Check sheet for the drawn part. Datum: minimum x, y, z corner. Units: mm. Give positions to 0.01 mm unless a question says otherwise; leave off trailing zeros. Order: outer loops, then holes, each group sorted by start corner. A loop starts at its lowest first (then second) coordinate and runs counter-clockwise, first axis right, second up. Notation, with made-up numbers: M 23.5,-27 L 69.5,-27 A20 ccw 69.5,12 Z; hole C 85,75 d3. An arc over 180 degrees is marked long. Answer as CSV lines item,"result". Start each with the question number.
Q1. Section check C-C, the plane x = 178.5. Record the boundary of the cut face in (y, z).
Q2. Section check A-A, the plane z = 23.5. Record the boundary of the cut face in (x, y), then the cut area to 3 significant figures.
Q3. Mould release check, pull along X, two halves, no side actions. Record for the marked faces 1, 2 and 3: +X half, -X half, draft (parallel to the pull), parting line (faces both ways), or undercut.
Q4. Thickness scan on line 1 (X direction, y = 7, z = 10.75); line 2 (X direction, y = 65.5, z = 21.75); line 3 (Z direction, x = 56, y = 56.5). Record the ranges inside material, lowest first.
Q5. Go/stop test with flat-tipped pins: pin 1 (1.5 mm diameter, centred on x = 38, z = 11.5, fed in from +Y); pin 2 (2.5 mm diameter, centred on y = 94, z = 7, fed in from +X); pin 3 (10 mm diameter, centred on x = 39, y = 91.5, fed in from +Z). Record where each tip stops, or that it passes through.
Q6. Section check B-B, the plane y = 39. Record the boundary of the cut face in (x, z), then the cut area to 3 significant figures.
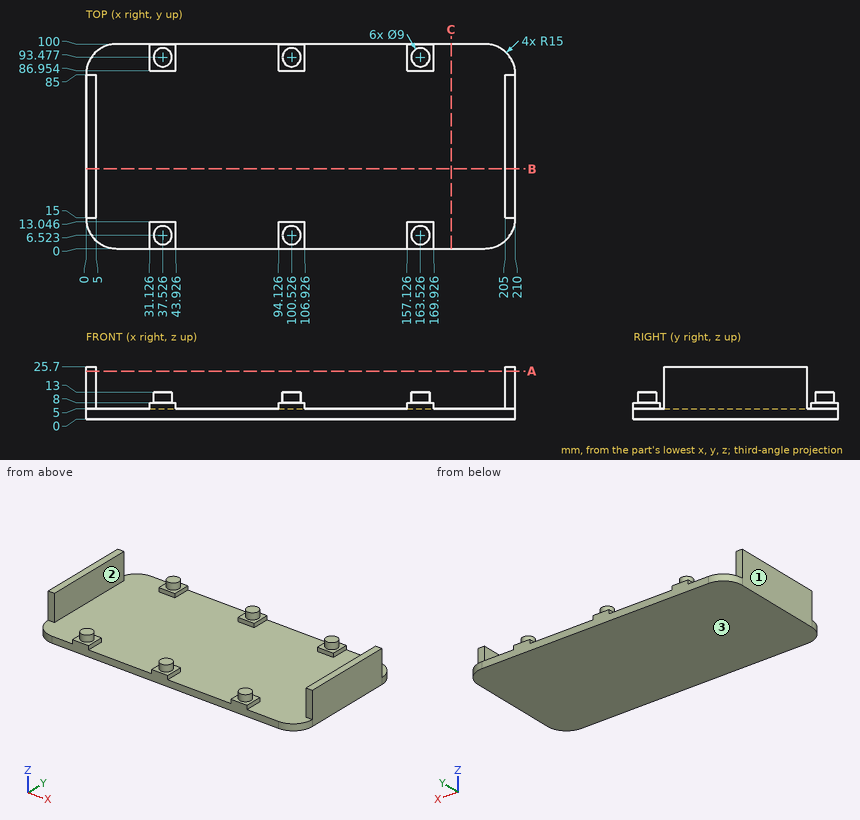
Answer block:
1,outline,"M 0,0 L 100,0 L 100,5 L 0,5 Z"
2,outline,"M 0,15 L 5,15 L 5,85 L 0,85 Z; M 205,15 L 210,15 L 210,85 L 205,85 Z"
2,area,"700 mm2"
3,face 1,"-X half"
3,face 2,"undercut"
3,face 3,"draft"
4,line 1,"x = 33.05 to 42, 96.05 to 105, 159.05 to 168"
4,line 2,"x = 0 to 5, 205 to 210"
4,line 3,"z = 0 to 5"
5,pin 1,"stops at y = 97.98"
5,pin 2,"stops at x = 169.93"
5,pin 3,"stops at z = 13"
6,outline,"M 0,0 L 210,0 L 210,25.7 L 205,25.7 L 205,5 L 5,5 L 5,25.7 L 0,25.7 Z"
6,area,"1,260 mm2"
